```python
from build123d import *

# Parameters (mm, degrees)
F1_DEPTH = 38.1
F3_DEPTH = 12.7
F5_DEPTH = 12.7


with BuildPart() as f1:
    # F0 (on Front) → F1 (new body)
    with BuildSketch(Plane.XZ):
        Polygon((0, 6.35), (0, 0), (25.4, 0), (25.4, 6.35), (19.05, 6.35), align=None)
        Polygon((0, 19.05), (0, 6.35), (19.05, 6.35), (19.05, 11.1125), (8.4666666667, 19.05), align=None)
        Polygon((19.05, 6.35), (25.4, 6.35), (19.05, 11.1125), align=None)
        Polygon((0, 25.4), (0, 19.05), (8.4666666667, 19.05), align=None)
    extrude(amount=F1_DEPTH)

    # F2 (on face) → F3 (cut)
    with BuildSketch(Plane.XZ.offset(38.1)):
        Polygon((0, 6.35), (25.4, 6.35), (0, 25.4), align=None)
    extrude(amount=-F3_DEPTH, mode=Mode.SUBTRACT)

    # F4 (on face) → F5 (cut)
    with BuildSketch(Plane.XZ.offset(25.4)):
        Polygon((0, 15.875), (12.7, 15.875), (0, 25.4), align=None)
    extrude(amount=-F5_DEPTH, mode=Mode.SUBTRACT)


solid = f1.part
```
Design review of the part built by this model. Coordinates are the model's own, in mm. A direction names the side the tool comes from. Coordinates: 2 decimals unless noted, no trailing zeros. Loops run counter-clockwise (first coordinate to the right, second up) from the corner with the lowest first, then second, coordinate; pieces in that order, holes last. Notation, with made-up numbers: M 67.5,67.25 L 72.5,67.25 A29 ccw 72.5,95.25 Z; hole C 52.25,-2.75 d5. An arc over 180 degrees is marked long. One line per question, with ' | ' between items.
(1) For pin 1 Ø8 at (x, y) = (3, -9) entering from +Z; pin 2 Ø8 at (x, y) = (11.5, -22) entering from +Z (3 decimals); pin 3 Ø1 at (x, y) = (7.5, -30.5) entering from +Z; pin 4 Ø7.5 at (x, z) = (7, 12) entering from -Y, all flat-tipped, find the tip position at first contact; note any pin that passes through.
Filled in:
pin 1: stops at z = 25.4 | pin 2: stops at z = 15.875 | pin 3: stops at z = 6.35 | pin 4: stops at y = -25.4
(2) Machinability: for faces 1 (the face through (3, -12.7, 19)), 2 (the face through (10, 0, 10)), which of the approach directions +Z, -Z, +X, -X, +Y, -Y give a long, thin tool a straight path to every point of the face, cutting with its end or side? Answer none if there is none.
Filled in:
face 1: +Z, +X, -X, -Y | face 2: +Z, -Z, +X, -X, +Y
(3) Wall thickness on probe 1 along Y at (x, z) = (14.5, 9.5); probe 2 along Z at (x, y) = (2.75, -21) (3 decimals); probe 3 along Y at (x, z) = (2, 18.25): over which ranges is each line inside the solid? List them lowest first.
Filled in:
probe 1: y = -25.4 to 0 | probe 2: z = 0 to 15.875 | probe 3: y = -12.7 to 0
(4) We need section C-C (z = 8.5). Give the boundary of the cut face in (x, y), and give its area (3 significant figures).
Filled in:
outline: M 0,-25.4 L 22.53,-25.4 L 22.53,0 L 0,0 Z | area: 572 mm^2
(5) We need section A-A (y = -8.5). Give the boundary of the cut face in (x, z).
Filled in:
outline: M 0,0 L 25.4,0 L 25.4,6.35 L 0,25.4 Z
